from build123d import *

# Parameters (mm, degrees)
SKETCH1_W           = 43.5
SKETCH1_H           = 21
SKETCH1_R           = 1.5
BOSS_EXTRUDE1_DEPTH = 1.5
SKETCH2_R           = 2.5
SKETCH2_W           = 10.433244148
SKETCH2_H           = 3.805065513
BOSS_EXTRUDE2_DEPTH = 10.5
SKETCH3_W           = 10.770790281
SKETCH3_H           = 10.218442062
BOSS_EXTRUDE3_DEPTH = 6
SKETCH4_W           = 9.543349793
SKETCH4_H           = 7.610131025
BOSS_EXTRUDE4_DEPTH = 5


with BuildPart() as part:
    # Sketch1 → Boss-Extrude1 (new body)
    with BuildSketch(Plane.XY):
        with Locations((21.75, 10.5)):
            Rectangle(SKETCH1_W, SKETCH1_H)
        with Locations((6.75, 18.7)):
            Circle(SKETCH1_R, mode=Mode.SUBTRACT)
        with Locations((36.75, 2.3)):
            Circle(SKETCH1_R, mode=Mode.SUBTRACT)
    extrude(amount=BOSS_EXTRUDE1_DEPTH)

    # Sketch2 → Boss-Extrude2 (add)
    with BuildSketch(Plane.XY.offset(1.5)):
        with Locations(Location((3.430450718, 9.165158469, 0), (0, 0, 180))):
            Circle(SKETCH2_R)
        with Locations(Location((38.013586465, 9.165158469, 0), (0, 0, 180))):
            Circle(SKETCH2_R)
        with Locations((13.37271867, 2.813153945)):
            Rectangle(SKETCH2_W, SKETCH2_H)
    extrude(amount=BOSS_EXTRUDE2_DEPTH)

    # Sketch3 → Boss-Extrude3 (add)
    with BuildSketch(Plane.XY.offset(1.5)):
        with Locations((16.057744738, 13.108311037)):
            Rectangle(SKETCH3_W, SKETCH3_H)
    extrude(amount=BOSS_EXTRUDE3_DEPTH)

    # Sketch4 → Boss-Extrude4 (add)
    with BuildSketch(Plane.XY.offset(1.5)):
        with Locations((27.902545446, 5.636267067)):
            Rectangle(SKETCH4_W, SKETCH4_H)
    extrude(amount=BOSS_EXTRUDE4_DEPTH)


solid = part.part
Here's how the part is built. I have some questions about the finished solid (model axes, mm). A direction names the side the tool comes from. Coordinates: 2 decimals unless noted, no trailing zeros. Write each loop counter-clockwise with the first axis right and the second up, starting at its lowest first coordinate (ties: lowest second). Pieces come first, ordered by that corner, then holes.
Item 1: Will these pins go through, and if not, where does the flat tip stop? pin 1 (3.5 mm diameter, centred on x = 6.75, y = 18.7, fed in from -Z); pin 2 (2.5 mm diameter, centred on x = 26, z = 3, fed in from +Y); pin 3 (2.5 mm diameter, centred on x = 36.75, y = 2.3, fed in from +Z); pin 4 (11 mm diameter, centred on x = 15, y = 11.5, fed in from +Z).
Item 2: I want a section at C-C on x = 6.75. Write out the boundary of the cut face in (y, z), and give its area (3 significant figures).
Item 3: I want a section at B-B on z = 2.75. Write out the boundary of the cut face in (x, y), and give its area (3 significant figures).
Item 4: I want a section at D-D on y = 6.25. Write out the boundary of the cut face in (x, z), and give its area (3 significant figures).
Item 5: If we mould it in two halves opening along X, with no side actions, what happens to faces 1 (the flat face through (43.5, 10, 1)), 2 (the flat face through (28, 6, 6.5)), 3 (the flat face through (13, 4.716, 7)), 4 (the cylindrical face through (40.51, 9.06, 6.68))? For each: +X half, -X half, draft (parallel to the pull), parting line (faces both ways), or undercut.
Item 6: If I drill on line 1 (Y direction, x = 6.75, z = 1.2); line 2 (Y direction, x = 36.75, z = 0.6); line 3 (X direction, y = 8.25, z = 4), over which ranges is the centre line in solid material (lowest first)?
Item 7: I want a section at A-A on y = 2.3. Write out the boundary of the cut face in (x, z), and give its area (3 significant figures).
Item 8: On a 3-axis mill with a long thin cutter (end or side, diameter ignored), from which of +Z, -Z, +X, -X, +Y, -Y can I reach the whole of each face in a straight line? I mean faces 5 (the flat face through (13, 0.911, 7)), 6 (the flat face through (32.674, 6, 4)), 7 (the flat face through (16, 13, 7.5)), 8 (the flat face through (16, 7.999, 4)), 9 (the flat face through (28, 1.831, 4)). Say none if no direction works.
Findings below:
1. pin 1: stops at z = 0
1. pin 2: stops at y = 9.44
1. pin 3: passes through
1. pin 4: stops at z = 7.5
2. outline: (0, 0) - (17.2, 0) - (17.2, 1.5) - (0, 1.5) - close; (20.2, 0) - (21, 0) - (21, 1.5) - (20.2, 1.5) - close
2. area: 27.0 mm2
3. outline: circle Ø5 at (3.43, 9.17); (8.16, 0.91) - (18.59, 0.91) - (18.59, 4.72) - (8.16, 4.72) - close; (10.67, 8) - (21.44, 8) - (21.44, 18.22) - (10.67, 18.22) - close; (23.13, 1.83) - (32.67, 1.83) - (32.67, 9.44) - (23.13, 9.44) - close; circle Ø5 at (38.01, 9.17)
3. area: 262 mm2
4. outline: (0, 0) - (43.5, 0) - (43.5, 1.5) - (32.67, 1.5) - (32.67, 6.5) - (23.13, 6.5) - (23.13, 1.5) - (0, 1.5) - close
4. area: 113 mm2
5. face 1: +X half
5. face 2: undercut
5. face 3: draft
5. face 4: undercut
6. line 1: y = 0 to 17.2, 20.2 to 21
6. line 2: y = 0 to 0.8, 3.8 to 21
6. line 3: x = 1.1 to 5.76, 10.67 to 21.44, 23.13 to 32.67, 35.69 to 40.34
7. outline: (0, 0) - (35.25, 0) - (35.25, 1.5) - (32.67, 1.5) - (32.67, 6.5) - (23.13, 6.5) - (23.13, 1.5) - (18.59, 1.5) - (18.59, 12) - (8.16, 12) - (8.16, 1.5) - (0, 1.5) - close; (38.25, 0) - (43.5, 0) - (43.5, 1.5) - (38.25, 1.5) - close
7. area: 218 mm2
8. face 5: +Z, +X, -X, -Y
8. face 6: +Z, +Y, -Y
8. face 7: +Z, +Y
8. face 8: +Z
8. face 9: +Z, +X, -Y
